The model under review builds one solid part; all positions refer to its coordinate system, in mm. Face numbers are marked on the shaded views. A direction names the side the tool comes from. Round coordinates to 2 decimals unless told otherwise and drop trailing zeros. Order: outer loops, then holes, each group sorted by start corner. A loop starts at its lowest first (then second) coordinate and runs counter-clockwise, first axis right, second up. Notation, with made-up numbers: (13, 78) - (31, 78) arc R6 ccw to (31, 85) - close; hole circle Ø3 at (88.25, 70.25). An arc over 180 degrees is marked (long way). One line per question, with ' | ' between items. Start each with the question number.
Item 1: Add section B-B on y = 24.5. State the section outline as (x, z) points.
Item 2: For L1, parallel to Z at x = -10.25, y = 40.5; L2, parallel to X at y = 38, z = 3.1; L3, parallel to X at y = 27.5, z = 2.9, list the stretches that pass through material, from the lowest coordinate up. Write a range as [from, to].
Item 3: Insertion check: pin 1 Ø2 at (x, z) = (-2, 3.5) entering from -Y; pin 2 Ø4 at (x, y) = (-3.5, 39.5) entering from +Z; pin 3 Ø2.5 at (x, y) = (-9, -33) entering from +Z. Each pin has a flat end and moves straight along its axis. Give the tip position at first contact, or say it passes through.
Item 4: Add section A-A on y = -18. State the section outline as (x, z) points, and give its area (3 significant figures).
Item 5: Tool access review of the marked faces 1 and 2: name each direction out of +Z, -Z, +X, -X, +Y, -Y from which nothing blocks a thin tool from reaching the whole face with its end or side.
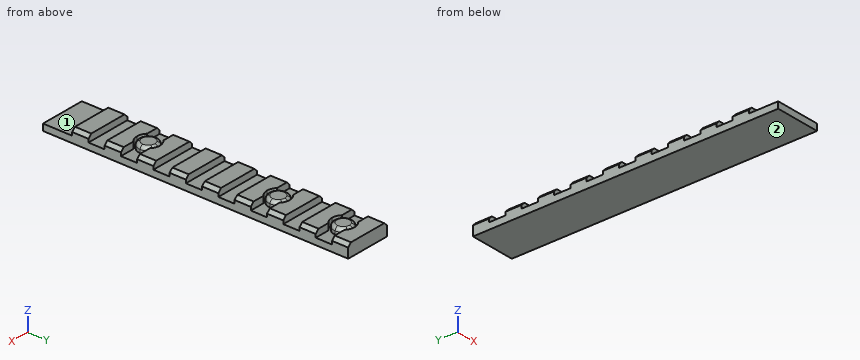
from build123d import *

# Parameters (mm, degrees)
F0_W     = 14
F0_H     = 94
F1_DEPTH = 2
F2_W     = 7
F2_H     = 5
F3_DEPTH = 2
F4_SIZE  = 1
F5_R     = 1


with BuildPart() as f1:
    # F0 (on Top) → F1 (new body)
    with BuildSketch(Plane.XY):
        with Locations((-7, 11.0699324605)):
            Rectangle(F0_W, F0_H)
    extrude(amount=F1_DEPTH)

    # F2 (on face) → F3 (join)
    with BuildSketch(Plane.XY.offset(2)):
        with BuildLine():
            Line((-7, 58.0699324605), (-14, 58.0699324605))
            Line((-14, 58.0699324605), (-14, 53.0699324605))
            Line((-14, 53.0699324605), (-9.4494897428, 53.0699324605))
            ThreePointArc((-9.4494897428, 53.0699324605), (-8.3228756555, 53.8103028097), (-7, 54.0699324605))
            Line((-7, 54.0699324605), (-7, 58.0699324605))
        make_face()
        with BuildLine():
            Line((0, 58.0699324605), (-7, 58.0699324605))
            Line((-7, 58.0699324605), (-7, 54.0699324605))
            ThreePointArc((-7, 54.0699324605), (-5.6771243445, 53.8103028097), (-4.5505102572, 53.0699324605))
            Line((-4.5505102572, 53.0699324605), (0, 53.0699324605))
            Line((0, 53.0699324605), (0, 58.0699324605))
        make_face()
        with BuildLine():
            Line((-9.4494897428, 48.0699324605), (-14, 48.0699324605))
            Line((-14, 48.0699324605), (-14, 43.0699324605))
            Line((-14, 43.0699324605), (-7, 43.0699324605))
            Line((-7, 43.0699324605), (-7, 47.0699324605))
            ThreePointArc((-7, 47.0699324605), (-8.3228756555, 47.3295621113), (-9.4494897428, 48.0699324605))
        make_face()
        with BuildLine():
            ThreePointArc((-4.5505102572, 48.0699324605), (-5.6771243445, 47.3295621113), (-7, 47.0699324605))
            Line((-7, 47.0699324605), (-7, 43.0699324605))
            Line((-7, 43.0699324605), (0, 43.0699324605))
            Line((0, 43.0699324605), (0, 48.0699324605))
            Line((0, 48.0699324605), (-4.5505102572, 48.0699324605))
        make_face()
        with BuildLine():
            Line((0, 38.0699324605), (-7, 38.0699324605))
            Line((-7, 38.0699324605), (-7, 34.0699324605))
            ThreePointArc((-7, 34.0699324605), (-5.6771243445, 33.8103028097), (-4.5505102572, 33.0699324605))
            Line((-4.5505102572, 33.0699324605), (0, 33.0699324605))
            Line((0, 33.0699324605), (0, 38.0699324605))
        make_face()
        with BuildLine():
            Line((-7, 38.0699324605), (-14, 38.0699324605))
            Line((-14, 38.0699324605), (-14, 33.0699324605))
            Line((-14, 33.0699324605), (-9.4494897428, 33.0699324605))
            ThreePointArc((-9.4494897428, 33.0699324605), (-8.3228756555, 33.8103028097), (-7, 34.0699324605))
            Line((-7, 34.0699324605), (-7, 38.0699324605))
        make_face()
        with BuildLine():
            Line((-9.4494897428, 28.0699324605), (-14, 28.0699324605))
            Line((-14, 28.0699324605), (-14, 23.0699324605))
            Line((-14, 23.0699324605), (-7, 23.0699324605))
            Line((-7, 23.0699324605), (-7, 27.0699324605))
            ThreePointArc((-7, 27.0699324605), (-8.3228756555, 27.3295621113), (-9.4494897428, 28.0699324605))
        make_face()
        with BuildLine():
            Line((0, 23.0699324605), (0, 28.0699324605))
            Line((0, 28.0699324605), (-4.5505102572, 28.0699324605))
            ThreePointArc((-4.5505102572, 28.0699324605), (-5.6771243445, 27.3295621113), (-7, 27.0699324605))
            Line((-7, 27.0699324605), (-7, 23.0699324605))
            Line((-7, 23.0699324605), (0, 23.0699324605))
        make_face()
        with Locations((-10.5, 15.5699324605)):
            Rectangle(F2_W, F2_H)
        with Locations((-3.5, 15.5699324605)):
            Rectangle(F2_W, F2_H)
        with Locations((-10.5, 5.5699324605)):
            Rectangle(F2_W, F2_H)
        with Locations((-3.5, 5.5699324605)):
            Rectangle(F2_W, F2_H)
        with BuildLine():
            Line((-7, -1.9300675395), (-14, -1.9300675395))
            Line((-14, -1.9300675395), (-14, -6.9300675395))
            Line((-14, -6.9300675395), (-9.4494897428, -6.9300675395))
            ThreePointArc((-9.4494897428, -6.9300675395), (-8.3228756555, -6.1896971903), (-7, -5.9300675395))
            Line((-7, -5.9300675395), (-7, -1.9300675395))
        make_face()
        with BuildLine():
            Line((0, -1.9300675395), (-7, -1.9300675395))
            Line((-7, -1.9300675395), (-7, -5.9300675395))
            ThreePointArc((-7, -5.9300675395), (-5.6771243445, -6.1896971903), (-4.5505102572, -6.9300675395))
            Line((-4.5505102572, -6.9300675395), (0, -6.9300675395))
            Line((0, -6.9300675395), (0, -1.9300675395))
        make_face()
        with BuildLine():
            Line((-9.4494897428, -11.9300675395), (-14, -11.9300675395))
            Line((-14, -11.9300675395), (-14, -16.9300675395))
            Line((-14, -16.9300675395), (-7, -16.9300675395))
            Line((-7, -16.9300675395), (-7, -12.9300675395))
            ThreePointArc((-7, -12.9300675395), (-8.3228756555, -12.6704378887), (-9.4494897428, -11.9300675395))
        make_face()
        with BuildLine():
            Line((0, -16.9300675395), (0, -11.9300675395))
            Line((0, -11.9300675395), (-4.5505102572, -11.9300675395))
            ThreePointArc((-4.5505102572, -11.9300675395), (-5.6771243445, -12.6704378887), (-7, -12.9300675395))
            Line((-7, -12.9300675395), (-7, -16.9300675395))
            Line((-7, -16.9300675395), (0, -16.9300675395))
        make_face()
        with Locations((-10.5, -24.4300675395)):
            Rectangle(F2_W, F2_H)
        with Locations((-3.5, -24.4300675395)):
            Rectangle(F2_W, F2_H)
        with BuildLine():
            Line((-7, 53.0699324605), (-8.5114243945, 53.0699324605))
            ThreePointArc((-8.5114243945, 53.0699324605), (-9.9213701751, 50.5699324605), (-8.5114243945, 48.0699324605))
            Line((-8.5114243945, 48.0699324605), (-7, 48.0699324605))
            Line((-7, 48.0699324605), (-7, 53.0699324605))
        make_face()
        with BuildLine():
            Line((-5.4885756055, 53.0699324605), (-7, 53.0699324605))
            Line((-7, 53.0699324605), (-7, 48.0699324605))
            Line((-7, 48.0699324605), (-5.4885756055, 48.0699324605))
            ThreePointArc((-5.4885756055, 48.0699324605), (-4.455414194, 49.1348412522), (-4.0786298249, 50.5699324605))
            ThreePointArc((-4.0786298249, 50.5699324605), (-4.455414194, 52.0050236688), (-5.4885756055, 53.0699324605))
        make_face()
        with BuildLine():
            ThreePointArc((-5.4885756055, 53.0699324605), (-6.2154688463, 53.3839890642), (-7, 53.4913026356))
            Line((-7, 53.4913026356), (-7, 53.0699324605))
            Line((-7, 53.0699324605), (-5.4885756055, 53.0699324605))
        make_face()
        with BuildLine():
            ThreePointArc((-7, 53.4913026356), (-7.7845311537, 53.3839890642), (-8.5114243945, 53.0699324605))
            Line((-8.5114243945, 53.0699324605), (-7, 53.0699324605))
            Line((-7, 53.0699324605), (-7, 53.4913026356))
        make_face()
        with BuildLine():
            Line((-7, 48.0699324605), (-8.5114243945, 48.0699324605))
            ThreePointArc((-8.5114243945, 48.0699324605), (-7.7845311537, 47.7558758567), (-7, 47.6485622853))
            Line((-7, 47.6485622853), (-7, 48.0699324605))
        make_face()
        with BuildLine():
            Line((-5.4885756055, 48.0699324605), (-7, 48.0699324605))
            Line((-7, 48.0699324605), (-7, 47.6485622853))
            ThreePointArc((-7, 47.6485622853), (-6.2154688463, 47.7558758567), (-5.4885756055, 48.0699324605))
        make_face()
        with BuildLine():
            Line((-7, 33.0699324605), (-7, 33.5699324605))
            ThreePointArc((-7, 33.5699324605), (-7.8660254038, 33.4422137837), (-8.6583123952, 33.0699324605))
            Line((-8.6583123952, 33.0699324605), (-7, 33.0699324605))
        make_face()
        with BuildLine():
            ThreePointArc((-5.3416876048, 33.0699324605), (-6.1339745962, 33.4422137837), (-7, 33.5699324605))
            Line((-7, 33.5699324605), (-7, 33.0699324605))
            Line((-7, 33.0699324605), (-5.3416876048, 33.0699324605))
        make_face()
        with BuildLine():
            Line((-5.3416876048, 33.0699324605), (-7, 33.0699324605))
            Line((-7, 33.0699324605), (-7, 28.0699324605))
            Line((-7, 28.0699324605), (-5.3416876048, 28.0699324605))
            ThreePointArc((-5.3416876048, 28.0699324605), (-4.3566179631, 29.151295295), (-4, 30.5699324605))
            ThreePointArc((-4, 30.5699324605), (-4.3566179631, 31.9885696259), (-5.3416876048, 33.0699324605))
        make_face()
        with BuildLine():
            Line((-7, 33.0699324605), (-8.6583123952, 33.0699324605))
            ThreePointArc((-8.6583123952, 33.0699324605), (-10, 30.5699324605), (-8.6583123952, 28.0699324605))
            Line((-8.6583123952, 28.0699324605), (-7, 28.0699324605))
            Line((-7, 28.0699324605), (-7, 33.0699324605))
        make_face()
        with BuildLine():
            Line((-7, 28.0699324605), (-8.6583123952, 28.0699324605))
            ThreePointArc((-8.6583123952, 28.0699324605), (-7.8660254038, 27.6976511372), (-7, 27.5699324605))
            Line((-7, 27.5699324605), (-7, 28.0699324605))
        make_face()
        with BuildLine():
            Line((-5.3416876048, 28.0699324605), (-7, 28.0699324605))
            Line((-7, 28.0699324605), (-7, 27.5699324605))
            ThreePointArc((-7, 27.5699324605), (-6.1339745962, 27.6976511372), (-5.3416876048, 28.0699324605))
        make_face()
        with BuildLine():
            Line((-7, -6.9300675395), (-7, -6.4300675395))
            ThreePointArc((-7, -6.4300675395), (-7.8660254038, -6.5577862163), (-8.6583123952, -6.9300675395))
            Line((-8.6583123952, -6.9300675395), (-7, -6.9300675395))
        make_face()
        with BuildLine():
            ThreePointArc((-5.3416876048, -6.9300675395), (-6.1339745962, -6.5577862163), (-7, -6.4300675395))
            Line((-7, -6.4300675395), (-7, -6.9300675395))
            Line((-7, -6.9300675395), (-5.3416876048, -6.9300675395))
        make_face()
        with BuildLine():
            Line((-5.3416876048, -6.9300675395), (-7, -6.9300675395))
            Line((-7, -6.9300675395), (-7, -11.9300675395))
            Line((-7, -11.9300675395), (-5.3416876048, -11.9300675395))
            ThreePointArc((-5.3416876048, -11.9300675395), (-4.3566179631, -10.848704705), (-4, -9.4300675395))
            ThreePointArc((-4, -9.4300675395), (-4.3566179631, -8.0114303741), (-5.3416876048, -6.9300675395))
        make_face()
        with BuildLine():
            Line((-7, -6.9300675395), (-8.6583123952, -6.9300675395))
            ThreePointArc((-8.6583123952, -6.9300675395), (-10, -9.4300675395), (-8.6583123952, -11.9300675395))
            Line((-8.6583123952, -11.9300675395), (-7, -11.9300675395))
            Line((-7, -11.9300675395), (-7, -6.9300675395))
        make_face()
        with BuildLine():
            Line((-7, -11.9300675395), (-8.6583123952, -11.9300675395))
            ThreePointArc((-8.6583123952, -11.9300675395), (-7.8660254038, -12.3023488628), (-7, -12.4300675395))
            Line((-7, -12.4300675395), (-7, -11.9300675395))
        make_face()
        with BuildLine():
            Line((-5.3416876048, -11.9300675395), (-7, -11.9300675395))
            Line((-7, -11.9300675395), (-7, -12.4300675395))
            ThreePointArc((-7, -12.4300675395), (-6.1339745962, -12.3023488628), (-5.3416876048, -11.9300675395))
        make_face()
    extrude(amount=F3_DEPTH)

    # F4
    f4_edges = [f1.edges().sort_by_distance(p)[0] for p in [
        (-14, 55.569932, 4),
        (-14, 45.569932, 4),
        (-14, 35.569932, 4),
        (-14, 25.569932, 4),
        (-14, 15.569932, 4),
        (-14, 5.569932, 4),
        (-14, -4.430068, 4),
        (-14, -14.430068, 4),
        (-14, -24.430068, 4),
        (0, -24.430068, 4),
        (0, -14.430068, 4),
        (0, -4.430068, 4),
        (0, 5.569932, 4),
        (0, 15.569932, 4),
        (0, 25.569932, 4),
        (0, 35.569932, 4),
        (0, 45.569932, 4),
        (0, 55.569932, 4),
    ]]
    chamfer(f4_edges, length=F4_SIZE)

    # F5
    f5_edges = [f1.edges().sort_by_distance(p)[0] for p in [
        (-5.341688, -11.930068, 4),
        (-5.341688, 28.069932, 4),
        (-5.488576, 53.069932, 4),
    ]]
    fillet(f5_edges, radius=F5_R)


solid = f1.part
Determined:
1) outline: (-14, 0) - (0, 0) - (0, 3) - (-1, 4) - (-13, 4) - (-14, 3) - close
2) L1: [0, 2] | L2: [-13.9, -0.1] | L3: [-14, -8.68], [-5.32, 0]
3) pin 1: y = -26.93 | pin 2: z = 4 | pin 3: z = 2
4) outline: (-14, 0) - (0, 0) - (0, 2) - (-14, 2) - close | area: 28.0 mm2
5) face 1: +Z, +X, -X, -Y | face 2: -Z, +X, -X, +Y, -Y
